from build123d import *

# Parameters (mm, degrees)
SKETCH1_W           = 101
SKETCH1_H           = 64
SKETCH1_R           = 1.5
BOSS_EXTRUDE1_DEPTH = 8
SKETCH2_W           = 8
SKETCH2_H           = 1
BOSS_EXTRUDE2_DEPTH = 101
FILLET1_R           = 5
SKETCH3_W           = 81
SKETCH3_H           = 19
CUT_EXTRUDE1_DEPTH  = 61.317907789
FILLET2_R           = 10
SKETCH4_W           = 34
SKETCH4_H           = 3
CUT_EXTRUDE2_DEPTH  = 114.204461043
FILLET3_START       = 39.83238
FILLET3_DEPTH       = 10.66762
FILLET3_START_2     = -50.5
FILLET3_2_DEPTH     = 10.012507722
FILLET3_START_3     = -40.487492278
FILLET3_3_DEPTH     = 9.987492378
FILLET3_START_4     = 30.4999999
FILLET3_4_DEPTH     = 9.3323801
FILLET3_START_5     = -1
FILLET3_5_DEPTH     = 4


with BuildPart() as part:
    # Sketch1 → Boss-Extrude1 (new body)
    with BuildSketch(Plane.XY):
        Rectangle(SKETCH1_W, SKETCH1_H)
        with Locations((-29, 24.5)):
            Circle(SKETCH1_R, mode=Mode.SUBTRACT)
        with Locations((29, 24.5)):
            Circle(SKETCH1_R, mode=Mode.SUBTRACT)
        with Locations((29, -24.5)):
            Circle(SKETCH1_R, mode=Mode.SUBTRACT)
        with Locations((-29, -24.5)):
            Circle(SKETCH1_R, mode=Mode.SUBTRACT)
        with Locations((45.5, -27)):
            Circle(SKETCH1_R, mode=Mode.SUBTRACT)
        with Locations((-45.5, 27)):
            Circle(SKETCH1_R, mode=Mode.SUBTRACT)
    extrude(amount=BOSS_EXTRUDE1_DEPTH)

    # Sketch2 → Boss-Extrude2 (add)
    with BuildSketch(Plane(origin=(-50.5, -4.5, 0), x_dir=(0, 1, 0), z_dir=(-1, 0, 0))):
        with Locations((21.5, 0.5)):
            Rectangle(SKETCH2_W, SKETCH2_H)
    extrude(amount=-BOSS_EXTRUDE2_DEPTH)

    # Fillet1
    fillet1_edges = [part.edges().sort_by_distance(p)[0] for p in [
        (50.5, -32, 4),
        (-50.5, -32, 4),
        (-50.5, 32, 4),
        (50.5, 32, 4),
    ]]
    fillet(fillet1_edges, radius=FILLET1_R)

    # Sketch3 → Cut-Extrude1 (cut, through all)
    with BuildSketch(Plane(origin=(0, 0, 0), x_dir=(-1, 0, 0), z_dir=(0, 0, -1))):
        with Locations((0, -7.5)):
            Rectangle(SKETCH3_W, SKETCH3_H)
    extrude(amount=-CUT_EXTRUDE1_DEPTH, mode=Mode.SUBTRACT)

    # Fillet2
    # the kernel refuses this fillet: 10 mm, written as the material it adds along each edge
    with BuildSketch(Plane(origin=(40.5, -17, 0), x_dir=(-1, 0, 0), z_dir=(0, 0, 1)), Plane(origin=(-40.5, -17, 0), x_dir=(0, 1, 0), z_dir=(0, 0, 1)), Plane(origin=(40.5, 2, 0), x_dir=(0, -1, 0), z_dir=(0, 0, 1))) as fillet2_piece_1:
        with BuildLine():
            CenterArc((FILLET2_R, -FILLET2_R), FILLET2_R, 90, 90)
            Line((0, -FILLET2_R), (0, 0))
            Line((0, 0), (FILLET2_R, 0))
        make_face()
    extrude(amount=8)
    with BuildSketch(Plane(origin=(-40.5, 2, 0), x_dir=(0, -1, 0), z_dir=(0, 0, 1))) as fillet2_piece_2:
        with BuildLine():
            CenterArc((FILLET2_R, FILLET2_R), FILLET2_R, 180, 90)
            Line((0, FILLET2_R), (0, 0))
            Line((0, 0), (FILLET2_R, 0))
        make_face()
    extrude(amount=8)

    # Sketch4 → Cut-Extrude2 (cut, through all)
    with BuildSketch(Plane(origin=(50.5, -18.5, 0), x_dir=(0, 1, 0), z_dir=(-1, 0, 0))):
        with Locations((3.5, -1.5)):
            Rectangle(SKETCH4_W, SKETCH4_H)
    extrude(amount=CUT_EXTRUDE2_DEPTH, mode=Mode.SUBTRACT)

    # Fillet3: read off the stored shape, not the designer's step
    # Fillet3 outline → Fillet3 (add)
    with BuildSketch(Plane.YZ.offset(FILLET3_START)):
        with BuildLine():
            Line((2, 3), (-5.141428429, 3))
            ThreePointArc((-5.141428429, 3), (-1.268444058, 2.219544027), (2.000001555, -1.587e-06))
            Line((2.000001555, -1.587e-06), (2, 3))
        make_face()
    extrude(amount=FILLET3_DEPTH)

    # Fillet3 2 outline → Fillet3 2 (add)
    with BuildSketch(Plane.YZ.offset(FILLET3_START_2)):
        with BuildLine():
            Line((2, 3), (-5.141428429, 3))
            ThreePointArc((-5.141428429, 3), (-1.268444058, 2.219544027), (2.000001555, -1.587e-06))
            Line((2.000001555, -1.587e-06), (2, 3))
        make_face()
    extrude(amount=FILLET3_2_DEPTH)

    # Fillet3 3 outline → Fillet3 3 (add)
    with BuildSketch(Plane.YZ.offset(FILLET3_START_3)):
        with BuildLine():
            Line((2, 3), (-5.141428429, 3))
            ThreePointArc((-5.141428429, 3), (-1.268444058, 2.219544027), (2.000001555, -1.587e-06))
            Line((2.000001555, -1.587e-06), (2, 3))
        make_face()
    extrude(amount=FILLET3_3_DEPTH)

    # Fillet3 4 outline → Fillet3 4 (add)
    with BuildSketch(Plane.YZ.offset(FILLET3_START_4)):
        with BuildLine():
            Line((2, 3), (-5.141428429, 3))
            ThreePointArc((-5.141428429, 3), (-1.268444058, 2.219544027), (2.000001555, -1.587e-06))
            Line((2.000001555, -1.587e-06), (2, 3))
        make_face()
    extrude(amount=FILLET3_4_DEPTH)

    # Fillet3 5 outline → Fillet3 5 (cut)
    with BuildSketch(Plane.XY.offset(FILLET3_START_5)):
        with BuildLine():
            Line((30.4999999, -7), (40.449874371, -7))
            ThreePointArc((40.449874371, -7), (37.208203932, -0.583801513), (30.5, 2))
            Line((30.5, 2), (30.4999999, -7))
        make_face()
        with BuildLine():
            Line((-40.449874371, -7), (-30.4999999, -7))
            Line((-30.4999999, -7), (-30.5, 2))
            ThreePointArc((-30.5, 2), (-37.208203932, -0.583801513), (-40.449874371, -7))
        make_face()
    extrude(amount=FILLET3_5_DEPTH, mode=Mode.SUBTRACT)


solid = part.part
Could you check a few things on this model? Use its own coordinates, in mm. A direction names the side the tool comes from. Coordinates: 2 decimals unless noted, no trailing zeros. Loops run counter-clockwise (first coordinate to the right, second up) from the corner with the lowest first, then second, coordinate; pieces in that order, holes last. Notation, with made-up numbers: (-1, 49) -> (54, 49) arc R24 cw to (54, 81) -> close; hole circle Ø6 at (71.5, 44). An arc over 180 degrees is marked (long way). Answer in a Markdown table with one row per item.
(1) If I drill on probe 1 along Y at (x, z) = (-29, 3.75); probe 2 along X at (y, z) = (-27, 6.95); probe 3 along Y at (x, z) = (45.5, 5.3), over which ranges is the centre line in solid material (lowest first)?
Results found:
| item | result |
|---|---|
| probe 1 | y = -32 to -26, -23 to -17, 2 to 23, 26 to 32 |
| probe 2 | x = -50.5 to 44, 47 to 50.5 |
| probe 3 | y = -32 to -28.5, -25.5 to 32 |
(2) Imagine slicing it at D-D (y = -1). List the corners of the cut face in (x, z) for me.
Results found:
| item | result |
|---|---|
| outline | (-50.5, 2.1) -> (-37.64, 2.1) -> (-37.64, 8) -> (-50.5, 8) -> close; (37.64, 2.1) -> (50.5, 2.1) -> (50.5, 8) -> (37.64, 8) -> close |
(3) Imagine slicing it at C-C (z = 5). List the corners of the cut face in (x, y) for me.
Results found:
| item | result |
|---|---|
| outline | (-50.5, -27) arc R5 ccw to (-45.5, -32) -> (45.5, -32) arc R5 ccw to (50.5, -27) -> (50.5, 27) arc R5 ccw to (45.5, 32) -> (-45.5, 32) arc R5 ccw to (-50.5, 27) -> close; hole circle Ø3 at (-45.5, 27); hole (-40.49, -7.5) arc R10 ccw to (-30.5, -17) -> (30.5, -17) arc R10 ccw to (40.49, -7.5) arc R10 ccw to (30.5, 2) -> (-30.5, 2) arc R10 ccw to start; hole circle Ø3 at (-29, -24.5); hole circle Ø3 at (-29, 24.5); hole circle Ø3 at (29, -24.5); hole circle Ø3 at (29, 24.5); hole circle Ø3 at (45.5, -27) |
(4) Imagine slicing it at B-B (x = -16). List the corners of the cut face in (y, z) for me.
Results found:
| item | result |
|---|---|
| outline | (-32, 3) -> (-17, 3) -> (-17, 8) -> (-32, 8) -> close; (2, 0) -> (13, 0) -> (13, -1) -> (21, -1) -> (21, 0) -> (32, 0) -> (32, 8) -> (2, 8) -> close |
(5) Thinking about a two-plate mould opening in X: for faces 4 (the face through (1, -22, 3)), 5 (the face through (27.89, -23.49, 5.46)), 6 (the face through (50.5, 6, 5)), 7 (the face through (-37.47, -14.17, 5.46)), which applies, released by +X, released by -X, zero draft, split by the parting line, or undercut?
Results found:
| item | result |
|---|---|
| face 4 | zero draft |
| face 5 | undercut |
| face 6 | released by +X |
| face 7 | undercut |
(6) Will these pins go through, and if not, where does the flat tip stop? pin 1 Ø8 at (x, y) = (-5.5, -18) entering from -Z; pin 2 Ø0.8 at (x, z) = (-4.5, -0.5) entering from +Y; pin 3 Ø3.5 at (x, y) = (1, 25.5) entering from -Z.
Results found:
| item | result |
|---|---|
| pin 1 | stops at z = 3 |
| pin 2 | stops at y = 21 |
| pin 3 | stops at z = 0 |
(7) Imagine slicing it at A-A (x = -29). List the corners of the cut face in (y, z) for me, plus the area to 3 significant figures.
Results found:
| item | result |
|---|---|
| outline | (-32, 3) -> (-26, 3) -> (-26, 8) -> (-32, 8) -> close; (-23, 3) -> (-17, 3) -> (-17, 8) -> (-23, 8) -> close; (2, 0) -> (13, 0) -> (13, -1) -> (21, -1) -> (21, 0) -> (23, 0) -> (23, 8) -> (2, 8) -> close; (26, 0) -> (32, 0) -> (32, 8) -> (26, 8) -> close |
| area | 284 mm^2 |
(8) For faces 1 (the face through (49, 30.57, 4.06)), 2 (the face through (1, 7, 0)), 3 (the face through (37.315, -14.319, 5.465)), which set-ups out of +Z, -Z, +X, -X, +Y, -Y let a thin tool reach every point of the face, with its end or its side?
Results found:
| item | result |
|---|---|
| face 1 | +Z, -Z, +X, +Y |
| face 2 | -Z, +X, -X, -Y |
| face 3 | +Z, -Z |
